Autodesk Fusion 360 part; units mm, degrees
sketch "Esquisse1" plane through (0, 0, 0) normal (0, 0, 1) x (1, 0, 0)
  line L0 (-8.5, 0) -> (8.5, 0)
  line L1 (8.5, 0) -> (8.5, -11)
  line L2 (8.5, -11) -> (-8.5, -11) construction
  line L3 (-8.5, -11) -> (-8.5, 0)
  circle A0 centre (0, 0) radius 3.5
  arc A1 (8.5, 0) -> (-8.5, 0) centre (0, 0) ccw
  line L4 (10.5, 0) -> (10.5, -13)
  line L5 (10.5, -13) -> (-10.5, -13)
  line L6 (-10.5, -13) -> (-10.5, 0)
  arc A2 (10.5, 0) -> (-10.5, 0) centre (0, 0) ccw
  line L7 (-8.5, -11) -> (-8.5, -13)
  line L8 (8.5, -11) -> (8.5, -13)
  line L9 (10.5, -13) -> (16.5, -13)
  line L10 (16.5, -13) -> (16.5, 0)
  line L11 (16.5, 0) -> (10.5, 0)
  line L12 (10.5, 0) -> (10.5, -13)
  line L13 (0, 0) -> (0, -13) construction
  line L14 (-16.5, -13) -> (-16.5, 0)
  line L15 (-10.5, -13) -> (-16.5, -13)
  line L16 (-16.5, 0) -> (-10.5, 0)
  circle A3 centre (13.5, -6.5) radius 1.7
  line L17 (16.5, -6.5) -> (10.5, -6.5) construction
  line L18 (13.5, 0) -> (13.5, -13) construction
  circle A4 centre (-13.5, -6.5) radius 1.7
  dimension "d1" = 17
  dimension "d2" = 17
  dimension "d3" = 11
  dimension "d4" = 7
  dimension "d5" = -2
  dimension "d6" = 6
  dimension "d7" = 3.4
extrude "Extrusion1" add sketch "Esquisse1" along normal blind 2 contours L4 L9 L10 L11 L12 | L6 L14 L15 L16 makes body 1 at (-13.4577, -11.3984, 0) makes body 2 at (13.5423, -11.3984, 0)
extrude "Extrusion2" add sketch "Esquisse1" along normal blind 9 contours L1 L3 A1 L4 L5 L6 A2 L7 L8 L12 bodies 1 2
sketch "Esquisse2" plane through (0, 0, 9) normal (0, 0, 1) x (-1, 0, 0)
  line L0 (8.5, 13) -> (8.5, 0)
  arc A0 (-8.5, 0) -> (8.5, 0) centre (0, 0) ccw
  line L1 (-8.5, 0) -> (-8.5, 13)
  line L2 (-8.5, 13) -> (-10.5, 13)
  line L3 (-10.5, 13) -> (-10.5, 0)
  arc A1 (-10.5, 0) -> (10.5, 0) centre (0, 0) ccw
  line L4 (10.5, 0) -> (10.5, 13)
  line L5 (10.5, 13) -> (8.5, 13)
  circle A2 centre (0, 0) radius 3.5
  line L6 (-10.5, 13) -> (10.5, 13)
  line L7 (10.5, 13) -> (10.5, 0)
  arc A3 (-10.5, 0) -> (10.5, 0) centre (0, 0) ccw
  line L8 (-10.5, 0) -> (-10.5, 13)
extrude "Extrusion3" add sketch "Esquisse2" along normal blind 2 bodies 1
fillet "Congé1" radius 1 2 edges at (10.5, -6.5, 2) (-10.5, -6.5, 2) on bodies 1
CAD build for the part. Positions are in the model's coordinates, mm. A direction names the side the tool comes from. Round coordinates to 2 decimals unless told otherwise and drop trailing zeros. Write each loop counter-clockwise with the first axis right and the second up, starting at its lowest first coordinate (ties: lowest second). Pieces come first, ordered by that corner, then holes.
Item 1: Drill centre lines: L1, parallel to X at y = -4.75, z = 1.75; L2, parallel to Y at x = 13.5, z = 1.15; L3, parallel to X at y = 0, z = 9.9. Where is each one in solid material? Low to high.
Filled in:
L1: x = -16.5 to -8.5, 8.5 to 16.5
L2: y = -13 to -8.2, -4.8 to 0
L3: x = -10.5 to -3.5, 3.5 to 10.5
Item 2: Band-saw the part on A-A on x = 0. Write the cut outline in (y, z), then the cut area to 3 significant figures.
Filled in:
outline: (-13, 9) - (-3.5, 9) - (-3.5, 11) - (-13, 11) - close; (3.5, 9) - (8.5, 9) - (8.5, 0) - (10.5, 0) - (10.5, 11) - (3.5, 11) - close
area: 51.0 mm2
Item 3: Tool access for faces 1 (the flat face through (-10.5, -7, 7)), 2 (the flat face through (0, -5, 9)), 3 (the flat face through (10.5, -7, 7)): list every direction of +Z, -Z, +X, -X, +Y, -Y with a clear straight run to the whole face (end or side of a thin tool).
Filled in:
face 1: +Z, -X, +Y, -Y
face 2: -Z, -Y
face 3: +Z, +X, +Y, -Y
Item 4: Band-saw the part on D-D on x = 13.5. Write the cut outline in (y, z).
Filled in:
outline: (-13, 0) - (-8.2, 0) - (-8.2, 2) - (-13, 2) - close; (-4.8, 0) - (0, 0) - (0, 2) - (-4.8, 2) - close
Item 5: Drop flat-ended pins along their axis: pin 1 Ø8.5 at (x, y) = (-2, 1) entering from -Z; pin 2 Ø1.5 at (x, y) = (-14.5, -8.5) entering from +Z; pin 3 Ø2 at (y, z) = (-6.5, 9) entering from +X; pin 4 Ø3 at (x, y) = (13.5, -6.5) entering from +Z (1 decimal). Give the stop position or say it passes through.
Filled in:
pin 1: stops at z = 9
pin 2: stops at z = 2
pin 3: stops at x = 10.5
pin 4: passes through
Item 6: Band-saw the part on C-C on z = 4.25. Write the cut outline in (x, y), then the cut area to 3 significant figures.
Filled in:
outline: (-10.5, -13) - (-8.5, -13) - (-8.5, 0) arc R8.5 cw to (8.5, 0) - (8.5, -13) - (10.5, -13) - (10.5, 0) arc R10.5 ccw to (-10.5, 0) - close
area: 112 mm2
Item 7: Band-saw the part on B-B on y = -2.5. Write the cut outline in (x, z).
Filled in:
outline: (-16.5, 0) - (-8.5, 0) - (-8.5, 9) - (-2.45, 9) - (-2.45, 11) - (-10.5, 11) - (-10.5, 3) arc R1 cw to (-11.5, 2) - (-16.5, 2) - close; (2.45, 9) - (8.5, 9) - (8.5, 0) - (16.5, 0) - (16.5, 2) - (11.5, 2) arc R1 cw to (10.5, 3) - (10.5, 11) - (2.45, 11) - close
Item 8: Mould opens along Y. For faces 4 (the flat face through (8.5, -6, 4)), 5 (the cylindrical face through (14.3, -5, 1)), 6 (the flat face through (1, -13, 10)) say: released by +Y, released by -Y, zero draft, split by the parting line, or undercut.
Filled in:
face 4: zero draft
face 5: undercut
face 6: released by -Y
